Read the model definition and answer for the solid it produces. Units are mm, in the model's axes. Face numbers are marked on the shaded views. A direction names the side the tool comes from. Give positions to 0.01 mm unless a question says otherwise; leave off trailing zeros. Loops run counter-clockwise (first coordinate to the right, second up) from the corner with the lowest first, then second, coordinate; pieces in that order, holes last. Notation, with made-up numbers: (-17, 83) - (2, 83) arc R10 ccw to (2, 93) - close; hole circle Ø2 at (-17, 42). An arc over 180 degrees is marked (long way). Use a Markdown table: item, result. Add a question column.
Item 1: Each of these flat-tipped pins is pushed along its axis until it touches: P1, Ø6, axis at x = 5.5, z = -23, coming from the +Y side; P2, Ø5.5, axis at y = 2, z = -2, coming from the -X side; P3, Ø3, axis at x = 1.5, z = -4, coming from the +Y side. Where does it stop, or does it pass through?
Item 2: A cutting plane is placed at A-A (y = 0). Determine the outline of the cut face in (x, z) (3 decimals).
Item 3: A cutting plane is placed at B-B (z = 0). Determine the outline of the cut face in (x, y) (3 decimals).
Item 4: Which of the six approach directions +Z, -Z, +X, -X, +Y, -Y give full straight-line access (tool end or side, diameter ignored) to the marked faces 1 and 2?
Item 5: A cutting plane is placed at D-D (z = -10.5). Determine the outline of the cut face in (x, y), plus the area to 3 significant figures.
Item 6: Consider probe 1 along Y at (x, z) = (-4.25, 0) (3 decimals); probe 2 along X at (y, z) = (0, 9); probe 3 along Y at (x, z) = (3, -18). Determine where each line is inside the solid, lowest interval first. Write a range as [from, to].
Item 7: For a pull along Y with two mould halves and no side action, classify the marked faces 3, 4 and 5 as +Y half, -Y half, draft (parallel to the pull), parting line (faces both ways), or undercut.
Item 8: A cutting plane is placed at C-C (z = -24.5). Determine the outline of the cut face in (x, y), plus the area to 3 significant figures.
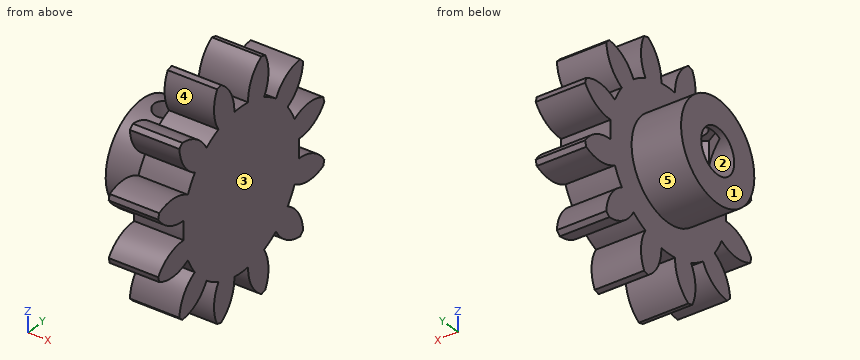
from build123d import *

# Parameters (mm, degrees)
BASPROSKE_W             = 12.7
BASPROSKE_H             = 29.633333333
TOOTHCUT_DEPTH          = 44.789940499
TEETHCUTS_COUNT         = 12
TEETHCUTS_ANGLE         = 330
SKETCH1_R               = 12.7
SKETCH1_R_2             = 5.715
BOSS_EXTRUDE1_DEPTH     = 12.7
CUT_EXTRUDE1_REACH      = 55.104
CUT_EXTRUDE1_END_RADIUS = 5.715
SKETCH2_R               = 3.2512
CUT_EXTRUDE2_DEPTH      = 7.62


with BuildPart() as part:
    # BasProSke → Base-Revolve (revolve)
    with BuildSketch(Plane(origin=(0, 0, 0), x_dir=(1, 0, 0), z_dir=(0, 1, 0)), mode=Mode.PRIVATE) as base_revolve_sk:
        with Locations((6.35, 14.816666667)):
            Rectangle(BASPROSKE_W, BASPROSKE_H)
    revolve(base_revolve_sk.sketch.rotate(Axis((-10, 0, 0), (1, 0, 0)), 180), axis=Axis((-10, 0, 0), (1, 0, 0)))

    # TooCutSke → ToothCut (cut, through all)
    with BuildSketch(Plane(origin=(0, 0, 0), x_dir=(0, 0, -1), z_dir=(1, 0, 0))):
        with BuildLine():
            ThreePointArc((2.3928109, 19.964179219), (0, 20.107063333), (-2.3928109, 19.964179219))
            ThreePointArc((-2.3928109, 19.964179219), (-3.536123556, 24.99754811), (-7.005125344, 28.819588509))
            ThreePointArc((-7.005125344, 28.819588509), (0, 29.658733333), (7.005125344, 28.819588509))
            ThreePointArc((7.005125344, 28.819588509), (3.536123556, 24.99754811), (2.3928109, 19.964179219))
        make_face()
    toothcut = extrude(amount=TOOTHCUT_DEPTH, mode=Mode.SUBTRACT)

    # TeethCuts: ToothCut ×12 about axis
    teethcuts_axis = Axis((-10, 0, 0), (1, 0, 0))
    for i in range(1, TEETHCUTS_COUNT):
        add(toothcut.rotate(teethcuts_axis, i * TEETHCUTS_ANGLE / (TEETHCUTS_COUNT - 1)), mode=Mode.SUBTRACT)

    # Sketch1 → Boss-Extrude1 (add)
    with BuildSketch(Plane.ZY):
        with Locations(Location((0, 0, 0), (0, 0, 180))):
            Circle(SKETCH1_R)
        Circle(SKETCH1_R_2, mode=Mode.SUBTRACT)
    extrude(amount=BOSS_EXTRUDE1_DEPTH)

    # Cut-Extrude1: up to this cylinder (the profile starts outside it)
    cut_extrude1_end = Plane(origin=(-6.35, 0, 0), z_dir=(1, 0, 0)) * Cylinder(CUT_EXTRUDE1_END_RADIUS, 122.638, mode=Mode.PRIVATE)
    # Sketch2 → Cut-Extrude1 (cut, up to the surface)
    with BuildSketch(Plane.XY.offset(13.97), mode=Mode.PRIVATE) as cut_extrude1_sk1:
        with Locations((-6.35, 0)):
            Circle(SKETCH2_R)
    cut_extrude1_tool1 = extrude(cut_extrude1_sk1.sketch, amount=-CUT_EXTRUDE1_REACH, mode=Mode.PRIVATE) - cut_extrude1_end
    add(cut_extrude1_tool1.solids().sort_by_distance((-6.35, 0, 13.97))[0], mode=Mode.SUBTRACT)

    # Sketch4 → Cut-Extrude2 (cut)
    with BuildSketch(Plane.XY):
        Polygon((-1.524, 2.786292399), (-6.35, 5.572584798), (-11.176, 2.786292399), (-11.176, -2.786292399), (-6.35, -5.572584798), (-1.524, -2.786292399), align=None)
    extrude(amount=CUT_EXTRUDE2_DEPTH, mode=Mode.SUBTRACT)


solid = part.part
Geometry says:
| question | item | result |
|---|---|---|
| 1 | P1 | y = 21.45 |
| 1 | P2 | x = 0 |
| 1 | P3 | y = 27.62 |
| 2 | outline | (-12.7, -12.7) - (0, -12.7) - (0, -20.107) - (12.7, -20.107) - (12.7, 20.107) - (0, 20.107) - (0, 12.7) - (-3.099, 12.7) - (-3.099, 7.62) - (-1.524, 7.62) - (-1.524, 5.715) - (0, 5.715) - (0, -5.715) - (-12.7, -5.715) - close; (-12.7, 5.715) - (-11.176, 5.715) - (-11.176, 7.62) - (-9.601, 7.62) - (-9.601, 12.7) - (-12.7, 12.7) - close |
| 3 | outline | (-12.7, -12.7) - (0, -12.7) - (0, -20.107) - (12.7, -20.107) - (12.7, 20.107) - (0, 20.107) - (0, 12.7) - (-12.7, 12.7) - (-12.7, 5.715) - (0, 5.715) - (0, -5.715) - (-12.7, -5.715) - close |
| 4 | face 1 | +Z, -Z, -X, +Y, -Y |
| 4 | face 2 | -X |
| 5 | outline | (-12.7, -7.14) - (0, -7.14) - (0, -17.15) - (12.7, -17.15) - (12.7, 17.15) - (0, 17.15) - (0, 7.14) - (-12.7, 7.14) - close |
| 5 | area | 617 mm² |
| 6 | probe 1 | [-12.7, -5.715], [5.715, 12.7] |
| 6 | probe 2 | [-12.7, -9.6], [-3.1, 12.7] |
| 6 | probe 3 | [-21.01, -13.37], [-8.96, 8.96], [13.37, 21.01] |
| 7 | face 3 | draft |
| 7 | face 4 | undercut |
| 7 | face 5 | parting line |
| 8 | outline | (0, -9.43) - (12.7, -9.43) - (12.7, -3.29) - (0, -3.29) - close; (0, 3.29) - (12.7, 3.29) - (12.7, 9.43) - (0, 9.43) - close |
| 8 | area | 156 mm² |
